```python
from build123d import *

# Parameters (mm, degrees)
BOX003_W          = 1.3
BOX003_H          = 3.3
BOX003_DEPTH      = 10
BOX002_W          = 1.3
BOX002_H          = 3.3
BOX002_DEPTH      = 10
CYLINDER004_R     = 1
CYLINDER004_DEPTH = 10
CYLINDER003_R     = 1
CYLINDER003_DEPTH = 10
CYLINDER001_R     = 2.5
CYLINDER001_DEPTH = 4
CYLINDER_R        = 5.9
CYLINDER_DEPTH    = 4
BOX001_W          = 11.8
BOX001_H          = 32.4
BOX001_DEPTH      = 2.5
BOX_W             = 11.8
BOX_H             = 22.5
BOX_DEPTH         = 22.7
SKETCH005_W       = 3.6
SKETCH005_H       = 1.2
POCKET001_DEPTH   = 3


with BuildPart() as cubo003:
    # Box003 → Box003 (new body)
    with BuildSketch(Plane(origin=(5.25, 25, 12), x_dir=(1, 0, 0), z_dir=(0, 0, 1))):
        with Locations((0.65, 1.65)):
            Rectangle(BOX003_W, BOX003_H)
    extrude(amount=BOX003_DEPTH)


with BuildPart() as obj1:
    # Box002 → Box002 (new body)
    with BuildSketch(Plane(origin=(5.25, -6, 12), x_dir=(1, 0, 0), z_dir=(0, 0, 1))):
        with Locations((0.65, 1.65)):
            Rectangle(BOX002_W, BOX002_H)
    extrude(amount=BOX002_DEPTH)

    # Fusion005: union Cubo003
    add(cubo003.part)


with BuildPart() as taladro2:
    # Cylinder004 → Cylinder004 (new body)
    with BuildSketch(Plane(origin=(5.9, 24.85, 11), x_dir=(1, 0, 0), z_dir=(0, 0, 1))):
        Circle(CYLINDER004_R)
    extrude(amount=CYLINDER004_DEPTH)


with BuildPart() as taladros001:
    # Cylinder003 → Cylinder003 (new body)
    with BuildSketch(Plane(origin=(5.9, -2.35, 11), x_dir=(1, 0, 0), z_dir=(0, 0, 1))):
        Circle(CYLINDER003_R)
    extrude(amount=CYLINDER003_DEPTH)

    # Fusion004: union Taladro2
    add(taladro2.part)

    # Fusion006: union obj1
    add(obj1.part)


with BuildPart() as cilindro001:
    # Cylinder001 → Cylinder001 (new body)
    with BuildSketch(Plane(origin=(5.9, 10.3, 22.7), x_dir=(1, 0, 0), z_dir=(0, 0, 1))):
        Circle(CYLINDER001_R)
    extrude(amount=CYLINDER001_DEPTH)


with BuildPart() as fusion001:
    # Cylinder → Cylinder (new body)
    with BuildSketch(Plane(origin=(5.9, 16.6, 22.7), x_dir=(1, 0, 0), z_dir=(0, 0, 1))):
        Circle(CYLINDER_R)
    extrude(amount=CYLINDER_DEPTH)

    # Fusion001: union Cilindro001
    add(cilindro001.part)


with BuildPart() as cubo001:
    # Box001 → Box001 (new body)
    with BuildSketch(Plane(origin=(0, -4.7, 15.9), x_dir=(1, 0, 0), z_dir=(0, 0, 1))):
        with Locations((5.9, 16.2)):
            Rectangle(BOX001_W, BOX001_H)
    extrude(amount=BOX001_DEPTH)


with BuildPart() as ranura_cable:
    # Box → Box (new body)
    with BuildSketch(Plane.XY):
        with Locations((5.9, 11.25)):
            Rectangle(BOX_W, BOX_H)
    extrude(amount=BOX_DEPTH)

    # Fusion: union Cubo001
    add(cubo001.part)

    # Fusion003: union Fusion001
    add(fusion001.part)

    # Cut: cut Taladros001
    add(taladros001.part, mode=Mode.SUBTRACT)


with BuildPart() as ranura_cable_1:
    # Cut placement: moved
    add(ranura_cable.part.moved(Location((-5.9, 0, 0))))

    # Sketch005 → Pocket001 (cut)
    with BuildSketch(Plane(origin=(-5.9, 22.5, 0), x_dir=(-1, 0, 0), z_dir=(0, 1, 0))):
        with Locations((-5.9, 5.1)):
            Rectangle(SKETCH005_W, SKETCH005_H)
    extrude(amount=-POCKET001_DEPTH, mode=Mode.SUBTRACT)


solid = ranura_cable_1.part
```
The model under review builds one solid part; all positions refer to its coordinate system, in mm. A direction names the side the tool comes from. Coordinates: 2 decimals unless noted, no trailing zeros. Write each loop counter-clockwise with the first axis right and the second up, starting at its lowest first coordinate (ties: lowest second). Pieces come first, ordered by that corner, then holes. Notation, with made-up numbers: (13.5, 33.25) - (38.5, 33.25) arc R9 ccw to (38.5, 37.25) - close; hole circle Ø3 at (80.5, -3). An arc over 180 degrees is marked (long way). Answer in a Markdown table with one row per item. Add a question column.
Q1. Draft analysis for pull direction Y (two halves, no side actions). For faces 5 (the face through (0.03, -1.35, 17.13)), 6 (the face through (-3, 27.7, 17)), 7 (the face through (-1.4, 25.1, 15.9)), 8 (the face through (-0.1, 7.8, 24.7)), state which applies: +Y half, -Y half, draft (parallel to the pull), parting line (faces both ways), or undercut.
Q2. Consider section B-B on z = 18. Give the boundary of the cut face in (x, y).
Q3. To check wall thickness, follow line 1 along X through (y, z) = (-2.35, 17.55); line 2 along Y through (x, z) = (0, 17.05); line 3 along Y through (x, z) = (0, 9.5). State the ranges of each line that lie inside material, in increasing order. Write a range as from..to.
Q4. Consider section A-A on y = 24.85. Give the boundary of the cut face in (x, z), then the cut area to 3 significant figures.
Q5. Clearance check with flat-ended pins moving along their axes: pin 1 (4 mm diameter, centred on x = 2, y = -2.5, fed in from -Z); pin 2 (1.5 mm diameter, centred on x = 0, y = 21, fed in from -Z); pin 3 (6 mm diameter, centred on x = -2.5, z = 4, fed in from +Y); pin 4 (0.6 mm diameter, centred on x = -1, z = 5, fed in from +Y). State where each tip first meets the part, or that it passes through.
Q6. Consider section C-C on x = -4. Give the boundary of the cut face in (y, z), then the cut area to 3 significant figures.
Q7. Consider section D-D on y = 4.5. Give the boundary of the cut face in (x, z).
Q8. For faces 1 (the face through (-5, 21, 22.7)), 2 (the face through (-0.65, -4, 17)), 3 (the face through (0, 22.5, 21)), 4 (the face through (1.8, 21, 5)), list the 3-axis set-ups (+Z, -Z, +X, -X, +Y, -Y) from which the entire face can be reached by the end or side of a thin tool; tool diameter is ignored.
Answers below:
| question | item | result |
|---|---|---|
| 1 | face 5 | undercut |
| 1 | face 6 | +Y half |
| 1 | face 7 | draft |
| 1 | face 8 | undercut |
| 2 | outline | (-5.9, -4.7) - (-0.65, -4.7) - (-0.65, -3.11) arc R1 cw (long way) to (0.65, -3.11) - (0.65, -4.7) - (5.9, -4.7) - (5.9, 27.7) - (0.65, 27.7) - (0.65, 25.61) arc R1 cw (long way) to (-0.65, 25.61) - (-0.65, 27.7) - (-5.9, 27.7) - close |
| 3 | line 1 | -5.9..-1, 1..5.9 |
| 3 | line 2 | -1.35..23.85 |
| 3 | line 3 | 0..22.5 |
| 4 | outline | (-5.9, 15.9) - (-1, 15.9) - (-1, 18.4) - (-5.9, 18.4) - close; (1, 15.9) - (5.9, 15.9) - (5.9, 18.4) - (1, 18.4) - close |
| 4 | area | 24.5 mm² |
| 5 | pin 1 | z = 15.9 |
| 5 | pin 2 | z = 0 |
| 5 | pin 3 | y = 22.5 |
| 5 | pin 4 | y = 19.5 |
| 6 | outline | (-4.7, 15.9) - (0, 15.9) - (0, 0) - (22.5, 0) - (22.5, 15.9) - (27.7, 15.9) - (27.7, 18.4) - (22.5, 18.4) - (22.5, 22.7) - (20.94, 22.7) - (20.94, 26.7) - (12.26, 26.7) - (12.26, 22.7) - (0, 22.7) - (0, 18.4) - (-4.7, 18.4) - close |
| 6 | area | 570 mm² |
| 7 | outline | (-5.9, 0) - (5.9, 0) - (5.9, 22.7) - (-5.9, 22.7) - close |
| 8 | face 1 | +Z, -X, +Y |
| 8 | face 2 | +Z, -Z, -Y |
| 8 | face 3 | +Z, +X, -X, +Y |
| 8 | face 4 | +Y |
